```python
from build123d import *

# Parameters (mm, degrees)
MODEL_R             = 5.5
BOSS_EXTRUDE1_DEPTH = 3
SKETCH2_R           = 8.05
CUT_EXTRUDE1_DEPTH  = 2


with BuildPart() as part:
    # Model → Boss-Extrude1 (new body)
    with BuildSketch(Plane.XY):
        with BuildLine():
            Line((-19.814466094, 53.465533906), (-28.535533906, 44.744466094))
            ThreePointArc((-28.535533906, 44.744466094), (-29.619397663, 43.12234935), (-30, 41.208932188))
            Line((-30, 41.208932188), (-30, 1.5))
            ThreePointArc((-30, 1.5), (-29.560660172, 0.439339828), (-28.5, 0))
            Line((-28.5, 0), (28.5, 0))
            ThreePointArc((28.5, 0), (29.560660172, 0.439339828), (30, 1.5))
            Line((30, 1.5), (30, 41.208932188))
            ThreePointArc((30, 41.208932188), (29.619397663, 43.12234935), (28.535533906, 44.744466094))
            Line((28.535533906, 44.744466094), (19.814466094, 53.465533906))
            ThreePointArc((19.814466094, 53.465533906), (18.19234935, 54.549397663), (16.278932188, 54.93))
            Line((16.278932188, 54.93), (-16.278932188, 54.93))
            ThreePointArc((-16.278932188, 54.93), (-18.19234935, 54.549397663), (-19.814466094, 53.465533906))
        make_face()
        with Locations((0, 32.43)):
            Circle(MODEL_R, mode=Mode.SUBTRACT)
        with BuildLine():
            Line((22.5, 8.63), (22.5, 15.43))
            ThreePointArc((22.5, 15.43), (20, 17.93), (17.5, 15.43))
            Line((17.5, 15.43), (17.5, 8.63))
            ThreePointArc((17.5, 8.63), (20, 6.13), (22.5, 8.63))
        make_face(mode=Mode.SUBTRACT)
        with BuildLine():
            Line((-22.5, 8.63), (-22.5, 15.43))
            ThreePointArc((-22.5, 15.43), (-20, 17.93), (-17.5, 15.43))
            Line((-17.5, 15.43), (-17.5, 8.63))
            ThreePointArc((-17.5, 8.63), (-20, 6.13), (-22.5, 8.63))
        make_face(mode=Mode.SUBTRACT)
        with BuildLine():
            Line((-2.5, 8.63), (-2.5, 15.43))
            ThreePointArc((-2.5, 15.43), (0, 17.93), (2.5, 15.43))
            Line((2.5, 15.43), (2.5, 8.63))
            ThreePointArc((2.5, 8.63), (0, 6.13), (-2.5, 8.63))
        make_face(mode=Mode.SUBTRACT)
    extrude(amount=BOSS_EXTRUDE1_DEPTH)

    # Sketch2 → Cut-Extrude1 (cut)
    with BuildSketch(Plane.XY.offset(3)):
        with Locations((0, 32.43)):
            Circle(SKETCH2_R)
    extrude(amount=-CUT_EXTRUDE1_DEPTH, mode=Mode.SUBTRACT)


solid = part.part
```
Verification items for the finished model (mm, model axes). A direction names the side the tool comes from. Round coordinates to 2 decimals unless told otherwise and drop trailing zeros. Write each loop counter-clockwise with the first axis right and the second up, starting at its lowest first coordinate (ties: lowest second). Pieces come first, ordered by that corner, then holes. Notation, with made-up numbers: (18, 7.25) -> (61, 7.25) arc R15 cw to (61, 28.25) -> close; hole circle Ø6 at (-7, 17.5). An arc over 180 degrees is marked (long way). Write each question's results on one line, items separated by ' | '.
Q1. Sectioned sample at A-A, the plane x = 0. Record the boundary of the cut face in (y, z).
Derived:
outline: (0, 0) -> (6.13, 0) -> (6.13, 3) -> (0, 3) -> close; (17.93, 0) -> (26.93, 0) -> (26.93, 1) -> (24.38, 1) -> (24.38, 3) -> (17.93, 3) -> close; (37.93, 0) -> (54.93, 0) -> (54.93, 3) -> (40.48, 3) -> (40.48, 1) -> (37.93, 1) -> close
Q2. Thickness scan on probe 1 along Y at (x, z) = (0, 0.7); probe 2 along Y at (x, z) = (0, 2); probe 3 along X at (y, z) = (8.5, 1.05). Record the ranges inside material, lowest first.
Derived:
probe 1: y = 0 to 6.13, 17.93 to 26.93, 37.93 to 54.93 | probe 2: y = 0 to 6.13, 17.93 to 24.38, 40.48 to 54.93 | probe 3: x = -30 to -22.5, -17.5 to -2.5, 2.5 to 17.5, 22.5 to 30
Q3. Draft check along Y on faces 1 (the face through (29.55, 0.43, 1.48)), 2 (the face through (-22.5, 12, 1)), 3 (the face through (0, 22, 0)), 4 (the face through (0, 54.93, 1)). Enter one of: released by +Y, released by -Y, zero draft, split by the parting line, or undercut.
Derived:
face 1: released by -Y | face 2: undercut | face 3: zero draft | face 4: released by +Y
Q4. Sectioned sample at D-D, the plane y = 32.43. Record the boundary of the cut face in (x, z), and give its area (3 significant figures).
Derived:
outline: (-30, 0) -> (-5.5, 0) -> (-5.5, 1) -> (-8.05, 1) -> (-8.05, 3) -> (-30, 3) -> close; (5.5, 0) -> (30, 0) -> (30, 3) -> (8.05, 3) -> (8.05, 1) -> (5.5, 1) -> close | area: 137 mm²
Q5. Sectioned sample at C-C, the plane z = 0.55. Record the boundary of the cut face in (x, y), and give its area (3 significant figures).
Derived:
outline: (-30, 1.5) arc R1.5 ccw to (-28.5, 0) -> (28.5, 0) arc R1.5 ccw to (30, 1.5) -> (30, 41.21) arc R5 ccw to (28.54, 44.74) -> (19.81, 53.47) arc R5 ccw to (16.28, 54.93) -> (-16.28, 54.93) arc R5 ccw to (-19.81, 53.47) -> (-28.54, 44.74) arc R5 ccw to (-30, 41.21) -> close; hole (-22.5, 8.63) arc R2.5 ccw to (-17.5, 8.63) -> (-17.5, 15.43) arc R2.5 ccw to (-22.5, 15.43) -> close; hole circle Ø11 at (0, 32.43); hole (-2.5, 8.63) arc R2.5 ccw to (2.5, 8.63) -> (2.5, 15.43) arc R2.5 ccw to (-2.5, 15.43) -> close; hole (17.5, 8.63) arc R2.5 ccw to (22.5, 8.63) -> (22.5, 15.43) arc R2.5 ccw to (17.5, 15.43) -> close | area: 2,900 mm²
Q6. Access from +Z, -Z, +X, -X, +Y, -Y to the whole of each face (thin tool, end or side, straight path). Record for faces 5 (the face through (0, 0, 1)), 6 (the face through (2, 27, 1)), 7 (the face through (19.95, 6.13, 1.48)).
Derived:
face 5: +Z, -Z, +X, -X, -Y | face 6: +Z | face 7: +Z, -Z
Q7. Go/stop test with a flat-tipped pin: pin 1 Ø8 at (x, y) = (-1.5, 30) entering from +Z. Record where the tip stops, or that it passes through.
Derived:
pin 1: stops at z = 1
Q8. Sectioned sample at B-B, the plane y = 12. Record the boundary of the cut face in (x, z), and give its area (3 significant figures).
Derived:
outline: (-30, 0) -> (-22.5, 0) -> (-22.5, 3) -> (-30, 3) -> close; (-17.5, 0) -> (-2.5, 0) -> (-2.5, 3) -> (-17.5, 3) -> close; (2.5, 0) -> (17.5, 0) -> (17.5, 3) -> (2.5, 3) -> close; (22.5, 0) -> (30, 0) -> (30, 3) -> (22.5, 3) -> close | area: 135 mm²
